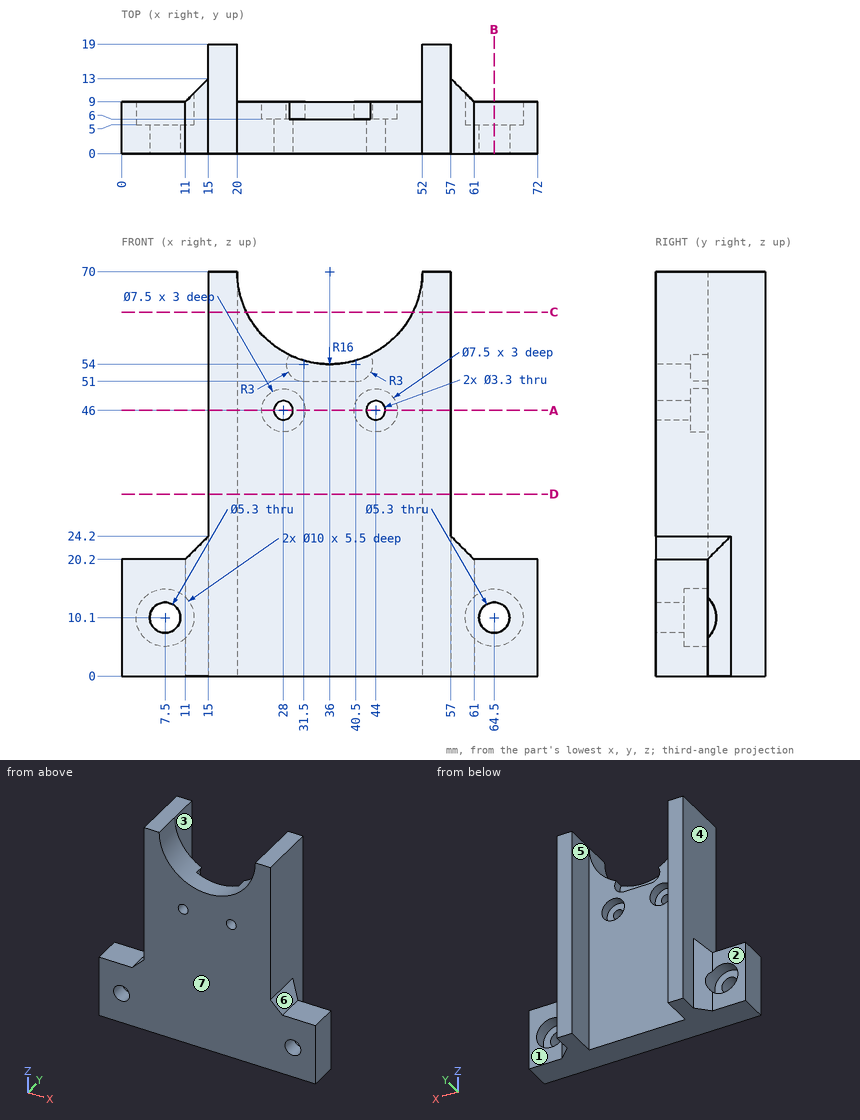
Could you check a few things on this drawing? It's one solid part, dimensions in mm from its lowest x, y, z. A direction names the side the tool comes from. Round coordinates to 2 decimals unless told otherwise and drop trailing zeros. Order: outer loops, then holes, each group sorted by start corner. A loop starts at its lowest first (then second) coordinate and runs counter-clockwise, first axis right, second up. Notation, with made-up numbers: M 85.5,72 L 96.5,72 A21 cw 96.5,100 Z; hole C 35.25,66.25 d1. An arc over 180 degrees is marked long. Return JSON: item names as keys, results as strings. Group by question number.
1. I'm going to push flat-ended pins straight in: pin 1 Ø12 at (x, z) = (6, 14) entering from +Y; pin 2 Ø4 at (y, z) = (9, 38) entering from -X; pin 3 Ø8 at (x, z) = (45, 45) entering from +Y. Where does each tip first touch, or does it pass through?
2. If we section it at C-C on z = 63: List the corners of the cut face in (x, y) for me.
3. If we mould it in two halves opening along X, with no side actions, what happens to the marked faces 5, 6 and 7? For each: pulls with the +X half, pulls with the -X half, needs draft (parallel to the pull), parting line crosses it, or undercut.
4. If we section it at D-D on z = 31.5: List the corners of the cut face in (x, y) for me, then the cut area to 3 significant figures.
5. On a 3-axis mill with a long thin cutter (end or side, diameter ignored), from which of +Z, -Z, +X, -X, +Y, -Y can I reach the whole of each face in a straight line? I mean the marked faces 1, 2, 3 and 4. Say none if no direction works.
6. Please list where these lines run through material, in increasing order: probe 1 along X at (y, z) = (3.5, 46); probe 2 along X at (y, z) = (3.9, 10.1); probe 3 along X at (y, z) = (13.5, 16).
7. If we section it at A-A on z = 46: List the corners of the cut face in (x, y) for me, then the cut area to 3 significant figures.
8. If we section it at B-B on x = 64.5: List the corners of the cut face in (y, z) for me.
Reply:
{
 "1": {"pin 1": "y = 10", "pin 2": "x = 15", "pin 3": "y = 9"},
 "2": {"outline": "M 15,0 L 21.61,0 L 21.61,9 L 20,9 L 20,19 L 15,19 Z; M 50.39,0 L 57,0 L 57,19 L 52,19 L 52,9 L 50.39,9 Z"},
 "3": {"face 5": "undercut", "face 6": "pulls with the +X half", "face 7": "needs draft"},
 "4": {"outline": "M 15,0 L 57,0 L 57,19 L 52,19 L 52,9 L 20,9 L 20,19 L 15,19 Z", "area": "478 mm^2"},
 "5": {"face 1": "+Z, -Z, +X, +Y", "face 2": "+Z, -Z, -X, +Y", "face 3": "+Z, -Z, +Y", "face 4": "+Z, -X, +Y"},
 "6": {"probe 1": "15 to 26.35, 29.65 to 42.35, 45.65 to 57", "probe 2": "0 to 4.85, 10.15 to 61.85, 67.15 to 72", "probe 3": "15 to 20, 52 to 57"},
 "7": {"outline": "M 15,0 L 26.35,0 L 26.35,6 L 24.25,6 L 24.25,9 L 20,9 L 20,19 L 15,19 Z; M 29.65,0 L 42.35,0 L 42.35,6 L 40.25,6 L 40.25,9 L 31.75,9 L 31.75,6 L 29.65,6 Z; M 45.65,0 L 57,0 L 57,19 L 52,19 L 52,9 L 47.75,9 L 47.75,6 L 45.65,6 Z", "area": "393 mm^2"},
 "8": {"outline": "M 0,0 L 9,0 L 9,5.1 L 5,5.1 L 5,7.45 L 0,7.45 Z; M 0,12.75 L 5,12.75 L 5,15.1 L 9,15.1 L 9,20.2 L 0,20.2 Z"}
}
